```python
from build123d import *

# Parameters (mm, degrees)
SKETCH2_R               = 350
BOSS_EXTRUDE1_DEPTH     = 1000
SKETCH3_R               = 20
BOSS_EXTRUDE2_DEPTH     = 30
BOSS_EXTRUDE3_DEPTH     = 100
SKETCH5_R               = 30
CUT_EXTRUDE1_DEPTH      = 351
CUT_EXTRUDE1_DEPTH_BACK = 351
SKETCH6_R               = 30
CUT_EXTRUDE2_DEPTH      = 351.000000102
CUT_EXTRUDE2_DEPTH_BACK = 29


with BuildPart() as part:
    # Sketch2 → Boss-Extrude1 (new body)
    with BuildSketch(Plane(origin=(0, 0, 0), x_dir=(1, 0, 0), z_dir=(0, 1, 0))):
        Circle(SKETCH2_R)
    extrude(amount=BOSS_EXTRUDE1_DEPTH)

    # Sketch3 → Boss-Extrude2 (add)
    with BuildSketch(Plane(origin=(0, 1000, 0), x_dir=(1, 0, 0), z_dir=(0, 1, 0))):
        with Locations((0, -84.841088142)):
            Circle(SKETCH3_R)
    extrude(amount=BOSS_EXTRUDE2_DEPTH)

    # Sketch4 → Boss-Extrude3 (add)
    with BuildSketch(Plane(origin=(0, 1000, 0), x_dir=(1, 0, 0), z_dir=(0, 1, 0))):
        Polygon((0, 134.555021266), (200, 134.555021266), (200, 287.228132327), (-200, 287.228132327), (-200, 134.555021266), align=None)
    extrude(amount=BOSS_EXTRUDE3_DEPTH)

    # Sketch5 → Cut-Extrude1 (cut, two sides)
    with BuildSketch(Plane.XY) as cut_extrude1_sk:
        with Locations((0, 876.38470429)):
            Circle(SKETCH5_R)
    extrude(amount=CUT_EXTRUDE1_DEPTH, mode=Mode.SUBTRACT)
    extrude(cut_extrude1_sk.sketch, amount=-CUT_EXTRUDE1_DEPTH_BACK, mode=Mode.SUBTRACT)

    # Sketch6 → Cut-Extrude2 (cut, two sides)
    with BuildSketch(Plane.XY) as cut_extrude2_sk:
        with Locations((0, 86.895276968)):
            Circle(SKETCH6_R)
    extrude(amount=CUT_EXTRUDE2_DEPTH, mode=Mode.SUBTRACT)
    extrude(cut_extrude2_sk.sketch, amount=-CUT_EXTRUDE2_DEPTH_BACK, mode=Mode.SUBTRACT)


solid = part.part
```
Could you check a few things on this model? Use its own coordinates, in mm. A direction names the side the tool comes from. Coordinates: 2 decimals unless noted, no trailing zeros. Order: outer loops, then holes, each group sorted by start corner. A loop starts at its lowest first (then second) coordinate and runs counter-clockwise, first axis right, second up. Notation, with made-up numbers: M 21,36.5 L 40,36.5 A34 ccw 40,75.5 Z; hole C -24,17 d1. An arc over 180 degrees is marked long. Use one line per item in the form item = value. Start each with the question number.
1. Please list where these lines run through material, in increasing order: line 1 (Y direction, x = 0, z = 83); line 2 (Y direction, x = 0, z = 177); line 3 (Y direction, x = 0, z = -184).
2. Suppose I cut it at D-D on x = -125. Write out the boundary of the cut face in (y, z).
3. For pin 1 (4 mm diameter, centred on y = 489.5, z = 127.5, fed in from -X); pin 2 (12 mm diameter, centred on x = -249, z = 196.5, fed in from -Y); pin 3 (3 mm diameter, centred on x = -241.5, y = 725.5, fed in from +Z); pin 4 (3 mm diameter, centred on x = 180, y = 502.5, fed in from +Z), each with a flat end and sliding along its axis, tell me the tip position at first contact or that it passes through.
4. Suppose I cut it at B-B on z = -248.5. Write out the boundary of the cut face in (x, y).
5. On a 3-axis mill with a long thin cutter (end or side, diameter ignored), from which of +Z, -Z, +X, -X, +Y, -Y can I reach the whole of each face in a straight line? I mean faces 1 (the cylindrical face through (-3.91, 116.64, 157.85)), 2 (the flat face through (200, 1049, -210)), 3 (the flat face through (0, 1030, 85)). Say none if no direction works.
6. We'd pull the mould along Y, two halves only. Please class faces 4 (the flat face through (3, 1049, -287.228)), 5 (the flat face through (0, 87, -29)), 6 (the flat face through (-3, 1100, -212)): +Y half, -Y half, draft (parallel to the pull), parting line (faces both ways), or undercut.
7. Suppose I cut it at A-A on x = 0. Write out the boundary of the cut face in (y, z).
8. Suppose I cut it at C-C on y = 591. Write out the boundary of the cut face in (x, z), then the cut area to 3 significant figures.
Geometry says:
q1.line_1 = 0 to 56.9, 116.9 to 846.38, 906.38 to 1030
q1.line_2 = 0 to 56.9, 116.9 to 846.38, 906.38 to 1000
q1.line_3 = 0 to 846.38, 906.38 to 1100
q2.outline = M 0,-326.92 L 1000,-326.92 L 1000,-287.23 L 1100,-287.23 L 1100,-134.56 L 1000,-134.56 L 1000,326.92 L 0,326.92 Z
q3.pin_1 = -326.73
q3.pin_2 = 0
q3.pin_3 = 254.75
q3.pin_4 = 301.06
q4.outline = M -246.47,0 L 246.47,0 L 246.47,1000 L 200,1000 L 200,1100 L -200,1100 L -200,1000 L -246.47,1000 Z; hole C 0,876.38 d60
q5.face_1 = +Z
q5.face_2 = +Z, -Z, +X, +Y
q5.face_3 = +Z, +X, -X, +Y
q6.face_4 = draft
q6.face_5 = undercut
q6.face_6 = +Y half
q7.outline = M 0,-350 L 846.38,-350 L 846.38,350 L 116.9,350 L 116.9,-29 L 56.9,-29 L 56.9,350 L 0,350 Z; M 906.38,-350 L 1000,-350 L 1000,-287.23 L 1100,-287.23 L 1100,-134.56 L 1000,-134.56 L 1000,64.84 L 1030,64.84 L 1030,104.84 L 1000,104.84 L 1000,350 L 906.38,350 Z
q8.outline = C 0,0 d700
q8.area = 385,000 mm^2
